Model file for the job. Use its own axes, mm. Face numbers are marked on the shaded views. A direction names the side the tool comes from. Coordinates: 2 decimals unless noted, no trailing zeros. Write each loop counter-clockwise with the first axis right and the second up, starting at its lowest first coordinate (ties: lowest second). Pieces come first, ordered by that corner, then holes. Notation, with made-up numbers: M 56,25.5 L 77,25.5 A26 ccw 77,42.5 Z; hole C -21,20 d6. An arc over 180 degrees is marked long. Answer in a Markdown table with one row per item. Add a question column.
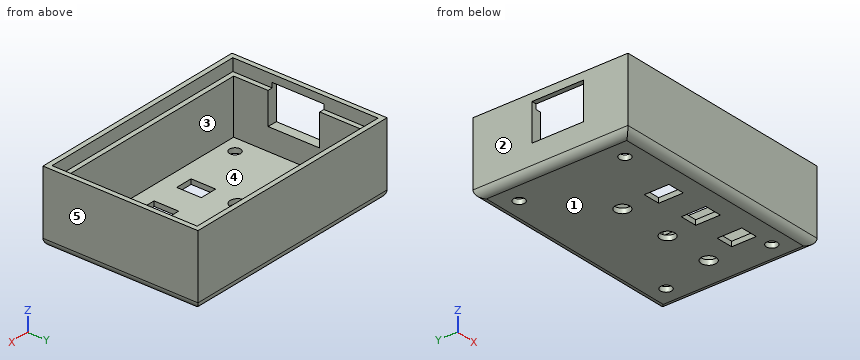
```python
from build123d import *

# Parameters (mm, degrees)
SKETCH3_W           = 92
SKETCH3_H           = 63
SKETCH3_R           = 3
SKETCH3_R_2         = 2.25
SKETCH3_W_2         = 7
SKETCH3_H_2         = 10
BOSS_EXTRUDE3_DEPTH = 29
SKETCH4_W           = 84
SKETCH4_H           = 55
CUT_EXTRUDE1_DEPTH  = 27
SKETCH5_W           = 88
SKETCH5_H           = 59
CUT_EXTRUDE2_DEPTH  = 5
FILLET1_R           = 3
SKETCH6_W           = 15
SKETCH6_H           = 21
CUT_EXTRUDE3_DEPTH  = 5


with BuildPart() as part:
    # Sketch3 → Boss-Extrude3 (new body)
    with BuildSketch(Plane.XY):
        with Locations((46, 31.5)):
            Rectangle(SKETCH3_W, SKETCH3_H)
        with Locations(Location((35, 31.5, 0), (0, 0, 180))):
            Circle(SKETCH3_R, mode=Mode.SUBTRACT)
        with Locations(Location((57, 31.5, 0), (0, 0, 180))):
            Circle(SKETCH3_R, mode=Mode.SUBTRACT)
        with Locations(Location((77, 31.5, 0), (0, 0, 180))):
            Circle(SKETCH3_R, mode=Mode.SUBTRACT)
        with Locations(Location((82, 53, 0), (0, 0, 180))):
            Circle(SKETCH3_R_2, mode=Mode.SUBTRACT)
        with Locations(Location((82, 10, 0), (0, 0, 180))):
            Circle(SKETCH3_R_2, mode=Mode.SUBTRACT)
        with Locations(Location((10.5, 10, 0), (0, 0, 180))):
            Circle(SKETCH3_R_2, mode=Mode.SUBTRACT)
        with Locations(Location((10.5, 53, 0), (0, 0, 180))):
            Circle(SKETCH3_R_2, mode=Mode.SUBTRACT)
        with Locations((71.5, 15.5)):
            Rectangle(SKETCH3_W_2, SKETCH3_H_2, mode=Mode.SUBTRACT)
        with Locations((54, 15.5)):
            Rectangle(SKETCH3_W_2, SKETCH3_H_2, mode=Mode.SUBTRACT)
        with Locations((36, 15.5)):
            Rectangle(SKETCH3_W_2, SKETCH3_H_2, mode=Mode.SUBTRACT)
    extrude(amount=BOSS_EXTRUDE3_DEPTH)

    # Sketch4 → Cut-Extrude1 (cut)
    with BuildSketch(Plane.XY.offset(29)):
        with Locations((46, 31.5)):
            Rectangle(SKETCH4_W, SKETCH4_H)
    extrude(amount=-CUT_EXTRUDE1_DEPTH, mode=Mode.SUBTRACT)

    # Sketch5 → Cut-Extrude2 (cut)
    with BuildSketch(Plane.XY.offset(29)):
        with Locations((46, 31.5)):
            Rectangle(SKETCH5_W, SKETCH5_H)
    extrude(amount=-CUT_EXTRUDE2_DEPTH, mode=Mode.SUBTRACT)

    # Fillet1
    fillet1_edges = [part.edges().sort_by_distance(p)[0] for p in [
        (0, 31.5, 0),
        (46, 63, 0),
        (92, 31.5, 0),
        (46, 0, 0),
    ]]
    fillet(fillet1_edges, radius=FILLET1_R)

    # Sketch6 → Cut-Extrude3 (cut)
    with BuildSketch(Plane.ZY):
        with Locations((18.5, 28.5)):
            Rectangle(SKETCH6_W, SKETCH6_H)
    extrude(amount=-CUT_EXTRUDE3_DEPTH, mode=Mode.SUBTRACT)


solid = part.part
```
1) Slice it at A-A (x = 70). Give the cut face in (y, z), then the cut area to 3 significant figures.
2) Slice it at D-D (y = 14.5). Give the cut face in (x, z).
3) Two-plate mould, pull along X, no slides. Class the marked faces 1, 2 and 3: released by +X, released by -X, zero draft, split by the parting line, or undercut.
4) Slice it at C-C (y = 35.5). Give the cut face in (x, z).
5) Flat gauge pins, fed straight in: pin 1 Ø2 at (y, z) = (18, 1) entering from -X; pin 2 Ø0.6 at (x, z) = (53.5, 0.5) entering from +Y; pin 3 Ø1 at (x, z) = (37.5, 1.5) entering from -Y. Where does each tip first touch, or does it go through?
6) Which spindle directions (+Z, -Z, +X, -X, +Y, -Y) get a long thin tool onto all of the face, cutting with end or side? Do the marked faces 4 and 5. Say none if no direction does.
7) Drill centre lines: probe 1 along Y at (x, z) = (70, 7.75); probe 2 along X at (y, z) = (31.5, 1.15); probe 3 along X at (y, z) = (31.5, 0.95). Where is each one in solid material? Low to high.
8) Slice it at B-B (x = 35). Give the cut face in (y, z).
Ans:
| question | item | result |
|---|---|---|
| 1 | outline | M 0,3 A3 ccw 3,0 L 10.5,0 L 10.5,2 L 4,2 L 4,24 L 2,24 L 2,29 L 0,29 Z; M 20.5,0 L 60,0 A3 ccw 63,3 L 63,29 L 61,29 L 61,24 L 59,24 L 59,2 L 20.5,2 Z |
| 1 | area | 298 mm2 |
| 2 | outline | M 0,3 A3 ccw 3,0 L 32.5,0 L 32.5,2 L 4,2 L 4,24 L 2,24 L 2,29 L 0,29 Z; M 39.5,0 L 50.5,0 L 50.5,2 L 39.5,2 Z; M 57.5,0 L 68,0 L 68,2 L 57.5,2 Z; M 75,0 L 89,0 A3 ccw 92,3 L 92,29 L 90,29 L 90,24 L 88,24 L 88,2 L 75,2 Z |
| 3 | face 1 | zero draft |
| 3 | face 2 | released by -X |
| 3 | face 3 | undercut |
| 4 | outline | M 0,3 A3 ccw 3,0 L 89,0 A3 ccw 92,3 L 92,29 L 90,29 L 90,24 L 88,24 L 88,2 L 4,2 L 4,11 L 0,11 Z; M 0,26 L 2,26 L 2,29 L 0,29 Z |
| 5 | pin 1 | stops at x = 0.17 |
| 5 | pin 2 | stops at y = 62.04 |
| 5 | pin 3 | stops at y = 0.17 |
| 6 | face 4 | +Z |
| 6 | face 5 | +Z, -Z, +X, +Y, -Y |
| 7 | probe 1 | y = 0 to 4, 59 to 63 |
| 7 | probe 2 | x = 0.64 to 32, 38 to 54, 60 to 74, 80 to 91.36 |
| 7 | probe 3 | x = 0.81 to 32, 38 to 54, 60 to 74, 80 to 91.19 |
| 8 | outline | M 0,3 A3 ccw 3,0 L 10.5,0 L 10.5,2 L 4,2 L 4,24 L 2,24 L 2,29 L 0,29 Z; M 20.5,0 L 28.5,0 L 28.5,2 L 20.5,2 Z; M 34.5,0 L 60,0 A3 ccw 63,3 L 63,29 L 61,29 L 61,24 L 59,24 L 59,2 L 34.5,2 Z |
